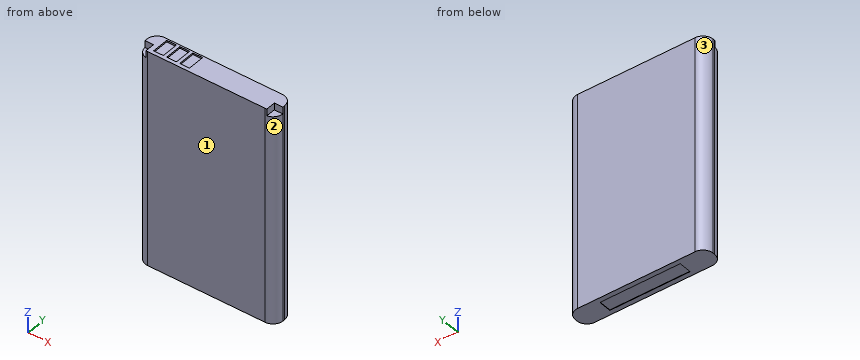
from build123d import *

# Parameters (mm, degrees)
SKETCH1_W           = 34
SKETCH1_H           = 53.2
BOSS_EXTRUDE1_DEPTH = 5.5
FILLET1_R           = 2.5
SKETCH2_W           = 2.4
SKETCH2_H           = 4.175
CUT_EXTRUDE1_DEPTH  = 0.4
LPATTERN1_COUNT     = 3
LPATTERN1_PITCH     = 3.22
SKETCH4_W           = 4.132195005
SKETCH4_H           = 2.4
CUT_EXTRUDE2_DEPTH  = 1.7
SKETCH5_W           = 19.8
SKETCH5_H           = 3.15
CUT_EXTRUDE3_DEPTH  = 0.1


with BuildPart() as part:
    # Sketch1 → Boss-Extrude1 (new body)
    with BuildSketch(Plane(origin=(0, 0, 0), x_dir=(1, 0, 0), z_dir=(0, 1, 0))):
        Rectangle(SKETCH1_W, SKETCH1_H)
    extrude(amount=BOSS_EXTRUDE1_DEPTH)

    # Fillet1
    fillet1_edges = [part.edges().sort_by_distance(p)[0] for p in [
        (-17, 5.5, 0),
        (17, 5.5, 0),
        (-17, 0, 0),
        (17, 0, 0),
    ]]
    fillet(fillet1_edges, radius=FILLET1_R)

    # Sketch2 → Cut-Extrude1 (cut)
    with BuildSketch(Plane.XY.offset(26.6)):
        with Locations((-12.5, 2.9875)):
            Rectangle(SKETCH2_W, SKETCH2_H)
    cut_extrude1 = extrude(amount=-CUT_EXTRUDE1_DEPTH, mode=Mode.SUBTRACT)

    # LPattern1: Cut-Extrude1 ×3
    with Locations(*[(i * LPATTERN1_PITCH, 0, 0) for i in range(1, LPATTERN1_COUNT)]):
        add(cut_extrude1, mode=Mode.SUBTRACT)

    # Sketch4 → Cut-Extrude2 (cut)
    with BuildSketch(Plane.XY.offset(26.6)):
        with Locations((-16.966097503, 1.2)):
            Rectangle(SKETCH4_W, SKETCH4_H)
    cut_extrude2 = extrude(amount=-CUT_EXTRUDE2_DEPTH, mode=Mode.SUBTRACT)

    # Mirror1: Cut-Extrude2 across plane
    add(cut_extrude2.mirror(Plane(origin=(0, 0, 0), x_dir=(0, 0, 1), z_dir=(1, 0, 0))), mode=Mode.SUBTRACT)

    # Sketch5 → Cut-Extrude3 (cut)
    with BuildSketch(Plane(origin=(0, 0, -26.6), x_dir=(-1, 0, 0), z_dir=(0, 0, -1))):
        with Locations((0, 2.75)):
            Rectangle(SKETCH5_W, SKETCH5_H)
    extrude(amount=-CUT_EXTRUDE3_DEPTH, mode=Mode.SUBTRACT)


solid = part.part
Geometry check sheet. Reference: the model listing, model coordinates, mm. Face numbers are marked on the shaded views. Round coordinates to 2 decimals unless told otherwise and drop trailing zeros. Loops run counter-clockwise (first coordinate to the right, second up) from the corner with the lowest first, then second, coordinate; pieces in that order, holes last.
Item 1: Mould release check, pull along X, two halves, no side actions. Record for the marked faces 1, 2 and 3: pulls with the +X half, pulls with the -X half, needs draft (parallel to the pull), parting line crosses it, or undercut.
Item 2: Gauge pin test, flat ends, axial feed: pin 1 (2.5 mm diameter, centred on x = -3, y = 3, fed in from -Z); pin 2 (0.6 mm diameter, centred on x = 15.5, y = 1.5, fed in from +Z); pin 3 (2.5 mm diameter, centred on x = -12.5, y = 3, fed in from +Z); pin 4 (0.8 mm diameter, centred on y = 1, z = 26, fed in from -X). Record the tip position at first contact, or that the pin passes through.
Item 3: Cross-section at A-A on z = 19.5. Record the boundary of the cut face in (x, y).
Item 4: Thickness scan on line 1 (Z direction, x = 4, y = 2.95); line 2 (Z direction, x = -5.5, y = 3.5); line 3 (X direction, y = 3.65, z = 7). Record the ranges inside material, lowest first.
Answer sheet:
1. face 1: needs draft
1. face 2: pulls with the +X half
1. face 3: pulls with the -X half
2. pin 1: stops at z = -26.5
2. pin 2: stops at z = 24.9
2. pin 3: stops at z = 26.6
2. pin 4: stops at x = -14.9
3. outline: (-17, 2.5) arc R2.5 ccw to (-14.5, 0) - (14.5, 0) arc R2.5 ccw to (17, 2.5) - (17, 3) arc R2.5 ccw to (14.5, 5.5) - (-14.5, 5.5) arc R2.5 ccw to (-17, 3) - close
4. line 1: z = -26.5 to 26.6
4. line 2: z = -26.5 to 26.2
4. line 3: x = -16.91 to 16.91
